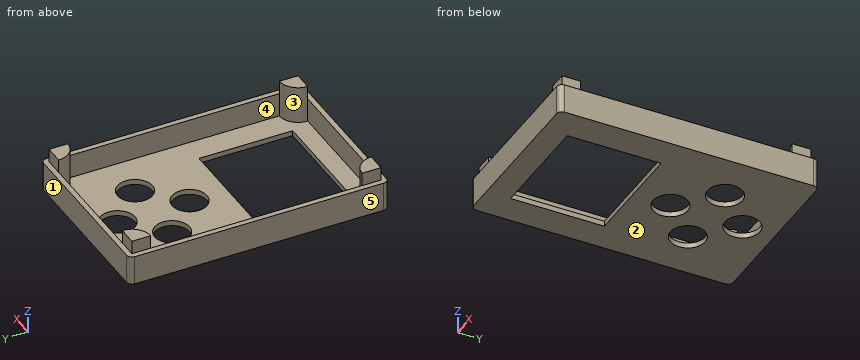
```python
from build123d import *

# Parameters (mm, degrees)
PAD001_DEPTH            = 11
SKETCH002_W             = 60
SKETCH002_H             = 93
POCKET001_DEPTH         = 9
SKETCH004_R             = 6.5
POCKET002_DEPTH         = 5
PAD002_DEPTH            = 14
BODY003_PLACEMENT_ANGLE = 180


with BuildPart() as part:
    # Sketch003 → Pad001 (new body)
    with BuildSketch(Plane.XY):
        with BuildLine():
            ThreePointArc((0, 2), (-1.414214, 1.414214), (-2, 0))
            Line((-2, 0), (-2, -93))
            ThreePointArc((-2, -93), (-1.414207, -94.414201), (0, -94.999981))
            Line((0, -94.999981), (60, -94.999981))
            ThreePointArc((60, -94.999981), (61.414214, -94.414194), (62, -92.999981))
            Line((62, 0), (62, -92.999981))
            ThreePointArc((62, 0), (61.414214, 1.414214), (60, 2))
            Line((0, 2), (60, 2))
        make_face()
    extrude(amount=PAD001_DEPTH)

    # Sketch002 (on Face10 of Pad001) → Pocket001 (cut)
    with BuildSketch(Plane.XY.offset(11)):
        with Locations((30, -46.5)):
            Rectangle(SKETCH002_W, SKETCH002_H)
    extrude(amount=-POCKET001_DEPTH, mode=Mode.SUBTRACT)

    # Sketch004 → Pocket002 (cut)
    with BuildSketch(Plane.XY):
        with Locations((30, -56)):
            Circle(SKETCH004_R)
        with Locations((43.435029, -69.435029)):
            Circle(SKETCH004_R)
        with Locations((16.564971, -69.435029)):
            Circle(SKETCH004_R)
        with Locations((30, -82.870058)):
            Circle(SKETCH004_R)
        Polygon((50.693539, -7), (50.693539, -42), (9.693539, -42), (9.693539, -7), (30.193539, -7), align=None)
    extrude(amount=POCKET002_DEPTH, mode=Mode.SUBTRACT)

    # Sketch006 (on Face24 of Pocket002) → Pad002 (join)
    with BuildSketch(Plane.XY.offset(2)):
        with BuildLine():
            Line((0, 0), (7, 0))
            ThreePointArc((0, -7), (4.949747, -4.949747), (7, 0))
            Line((0, -7), (0, 0))
        make_face()
        with BuildLine():
            Line((60, 0), (53, 0))
            ThreePointArc((53, 0), (55.050253, -4.949747), (60, -7))
            Line((60, 0), (60, -7))
        make_face()
        with BuildLine():
            Line((0, -93), (0, -86))
            ThreePointArc((7, -93), (4.949747, -88.050253), (0, -86))
            Line((0, -93), (7, -93))
        make_face()
        with BuildLine():
            Line((60, -93), (60, -86))
            ThreePointArc((60, -86), (55.050253, -88.050253), (53, -93))
            Line((60, -93), (53, -93))
        make_face()
    extrude(amount=PAD002_DEPTH)


with BuildPart() as part_1:
    # Body003 placement: moved
    add(part.part.moved(Location((-10, -93, 0))).rotate(Axis((-10, -93, 0), (0, 0, 1)), BODY003_PLACEMENT_ANGLE))


solid = part_1.part
```
Work out the finished part from the listing and answer in its coordinate system (mm). Face numbers are marked on the shaded views. A direction names the side the tool comes from. Give positions to 0.01 mm unless a question says otherwise; leave off trailing zeros. Order: outer loops, then holes, each group sorted by start corner. A loop starts at its lowest first (then second) coordinate and runs counter-clockwise, first axis right, second up.
1. Each of these flat-tipped pins is pushed along its axis until it touches: P1, Ø4, axis at y = -3, z = 14.5, coming from the +X side; P2, Ø5.5, axis at x = -14, z = 14.5, coming from the +Y side; P3, Ø2.5, axis at y = -5, z = 12.5, coming from the -X side; P4, Ø8, axis at x = -40, y = -10.13, coming from the +Z side. Where does it stop, or does it pass through?
Result sheet:
P1: stops at x = -10
P2: stops at y = 0
P3: stops at x = -70
P4: passes through
2. Section A-A, the plane x = -40 is taken. Determine the outline of the cut face in (y, z).
Result sheet:
outline: (-95, 0) - (-86, 0) - (-86, 2) - (-93, 2) - (-93, 11) - (-95, 11) - close; (-51, 0) - (-43.5, 0) - (-43.5, 2) - (-51, 2) - close; (-30.5, 0) - (-16.63, 0) - (-16.63, 2) - (-30.5, 2) - close; (-3.63, 0) - (2, 0) - (2, 11) - (0, 11) - (0, 2) - (-3.63, 2) - close
3. For the marked faces 4 and 5, determine the directions among +Z, -Z, +X, -X, +Y, -Y from which every point of the face is accessible in a straight line to the end or side of a thin tool.
Result sheet:
face 4: +Z
face 5: +Z, -Z, -X, +Y, -Y
4. Section D-D, the plane x = -23 is taken. Determine the outline of the cut face in (y, z).
Result sheet:
outline: (-95, 0) - (-86, 0) - (-86, 2) - (-93, 2) - (-93, 11) - (-95, 11) - close; (-51, 0) - (-29, 0) - (-29, 2) - (-51, 2) - close; (-18.13, 0) - (2, 0) - (2, 11) - (0, 11) - (0, 2) - (-18.13, 2) - close
5. Section C-C, the plane z = 9.75 is taken. Determine the outline of the cut face in (x, y), and give its area (3 significant figures).
Result sheet:
outline: (-72, -93) arc R2 ccw to (-70, -95) - (-10, -95) arc R2 ccw to (-8, -93) - (-8, 0) arc R2 ccw to (-10, 2) - (-70, 2) arc R2 ccw to (-72, 0) - close; hole (-70, -86) arc R7 cw to (-63, -93) - (-17, -93) arc R7 cw to (-10, -86) - (-10, -7) arc R7 cw to (-17, 0) - (-63, 0) arc R7 cw to (-70, -7) - close
area: 779 mm2
6. Straight lines are drawn through the part: L1, parallel to Y at x = -40, z = 1.2; L2, parallel to X at y = -16, z = 6; L3, parallel to Y at x = -22, z = 2.5. For each, find the intervals that lie inside material, in ascending order.
Result sheet:
L1: y = -95 to -86, -51 to -43.5, -30.5 to -16.63, -3.63 to 2
L2: x = -72 to -70, -10 to -8
L3: y = -95 to -93, 0 to 2
7. Section B-B, the plane y = -37 is taken. Determine the outline of the cut face in (x, z).
Result sheet:
outline: (-72, 0) - (-46.5, 0) - (-46.5, 2) - (-70, 2) - (-70, 11) - (-72, 11) - close; (-33.5, 0) - (-8, 0) - (-8, 11) - (-10, 11) - (-10, 2) - (-33.5, 2) - close
8. The mould has two halves that part along Y. Classify the marked faces 1, 2 and 3: released by +Y, released by -Y, zero draft, split by the parting line, or undercut.
Result sheet:
face 1: released by +Y
face 2: zero draft
face 3: undercut
